CAD build for the part. Positions are in the model's coordinates, mm. A direction names the side the tool comes from. Give positions to 0.01 mm unless a question says otherwise; leave off trailing zeros. Loops run counter-clockwise (first coordinate to the right, second up) from the corner with the lowest first, then second, coordinate; pieces in that order, holes last.
Item 1: Mould opens along X. For faces 3 (the flat face through (2, 0, 182)), 4 (the flat face through (143.29, 1.57, -95.33)), 5 (the cylindrical face through (88.43, 1.61, 171.83)) say: released by +X, released by -X, zero draft, split by the parting line, or undercut.
Item 2: Saw through at A-A on z = 109. Give the cut face in (x, y) (3 decimals).
Item 3: Saw through at B-B on z = -55.5. Give the cut face in (x, y) (3 decimals).
Item 4: Saw through at C-C on y = 1.5. Give the number of separate pieces and of enclosed holes in the cut face, plus the area to 3 significant figures.
Item 5: Which spindle directions (+Z, -Z, +X, -X, +Y, -Y) get a long thin tool onto all of the face, cutting with end or side? Do faces 1 (the cylindrical face through (-123.61, 1.61, 136.65)), 2 (the flat face through (2, 3.175, 182)). Say none if no direction does.
Item 6: Probe probe 1 along Z at (x, y) = (-66.5, 1.1); probe 2 along Z at (x, y) = (30, 0.2); probe 3 along Z at (x, y) = (42.5, 0.75). List the from-to ranges inside material, lowest first.
from build123d import *

# Parameters (mm, degrees)
BOSS_EXTRUDE1_DEPTH = 3.175
CUT_EXTRUDE1_DEPTH  = 252.960239461
SKETCH4_R           = 2.159
CUT_EXTRUDE2_DEPTH  = 252.960239461


with BuildPart() as part:
    # Sketch1 → Boss-Extrude1 (new body)
    with BuildSketch(Plane(origin=(0, 0, 0), x_dir=(1, 0, 0), z_dir=(0, 1, 0))):
        Polygon((-152.4, 86.220142619), (-134.439487758, 104.180654861), (134.439487758, 104.180654861), (152.4, 86.220142619), (152.4, -182.658832897), (134.439487758, -200.619345139), (-134.439487758, -200.619345139), (-152.4, -182.658832897), align=None)
    extrude(amount=BOSS_EXTRUDE1_DEPTH)

    # Sketch2 → Cut-Extrude1 (cut, through all)
    with BuildSketch(Plane(origin=(0, 3.175, 0), x_dir=(1, 0, 0), z_dir=(0, 1, 0))):
        with BuildLine():
            Line((-76.2, 78.780654861), (76.2, 78.780654861))
            ThreePointArc((76.2, 78.780654861), (88.275474207, 75.463786622), (98.518463274, 68.259630377))
            Line((98.518463274, 68.259630377), (116.478975516, 50.299118134))
            ThreePointArc((116.478975516, 50.299118134), (123.683131761, 40.056129068), (127, 27.980654861))
            Line((127, 27.980654861), (127, -124.419345139))
            ThreePointArc((127, -124.419345139), (123.683131761, -136.494819346), (116.478975516, -146.737808413))
            Line((116.478975516, -146.737808413), (98.518463274, -164.698320655))
            ThreePointArc((98.518463274, -164.698320655), (88.275474207, -171.9024769), (76.2, -175.219345139))
            Line((76.2, -175.219345139), (-76.2, -175.219345139))
            ThreePointArc((-76.2, -175.219345139), (-88.275474207, -171.9024769), (-98.518463274, -164.698320655))
            Line((-98.518463274, -164.698320655), (-116.478975516, -146.737808413))
            ThreePointArc((-116.478975516, -146.737808413), (-123.683131761, -136.494819346), (-127, -124.419345139))
            Line((-127, -124.419345139), (-127, 27.980654861))
            ThreePointArc((-127, 27.980654861), (-123.683131761, 40.056129068), (-116.478975516, 50.299118134))
            Line((-116.478975516, 50.299118134), (-98.518463274, 68.259630377))
            ThreePointArc((-98.518463274, 68.259630377), (-88.275474207, 75.463786622), (-76.2, 78.780654861))
        make_face()
    extrude(amount=-CUT_EXTRUDE1_DEPTH, mode=Mode.SUBTRACT)

    # Sketch4 → Cut-Extrude2 (cut, through all)
    with BuildSketch(Plane(origin=(0, 3.175, 0), x_dir=(1, 0, 0), z_dir=(0, 1, 0))):
        with Locations(Location((0, 92.750654861, 0), (0, 0, 270))):
            Circle(SKETCH4_R)
        with Locations(Location((-44.45, 92.750654861, 0), (0, 0, 270))):
            Circle(SKETCH4_R)
        with Locations(Location((44.45, 92.750654861, 0), (0, 0, 270))):
            Circle(SKETCH4_R)
        with Locations(Location((-22.225, 92.750654861, 0), (0, 0, 270))):
            Circle(SKETCH4_R)
        with Locations(Location((22.225, 92.750654861, 0), (0, 0, 270))):
            Circle(SKETCH4_R)
        with Locations(Location((-140.97, -48.219345139, 0), (0, 0, 270))):
            Circle(SKETCH4_R)
        with Locations(Location((-140.97, -25.994345139, 0), (0, 0, 270))):
            Circle(SKETCH4_R)
        with Locations(Location((-140.97, -3.769345139, 0), (0, 0, 270))):
            Circle(SKETCH4_R)
        with Locations(Location((140.97, -48.219345139, 0), (0, 0, 270))):
            Circle(SKETCH4_R)
        with Locations(Location((140.97, -25.994345139, 0), (0, 0, 270))):
            Circle(SKETCH4_R)
        with Locations(Location((140.97, -3.769345139, 0), (0, 0, 270))):
            Circle(SKETCH4_R)
        with Locations(Location((140.97, -92.669345139, 0), (0, 0, 90))):
            Circle(SKETCH4_R)
        with Locations(Location((140.97, -70.444345139, 0), (0, 0, 90))):
            Circle(SKETCH4_R)
        with Locations(Location((-140.97, -92.669345139, 0), (0, 0, 90))):
            Circle(SKETCH4_R)
        with Locations(Location((-140.97, -70.444345139, 0), (0, 0, 90))):
            Circle(SKETCH4_R)
        with Locations(Location((22.225, -189.189345139, 0), (0, 0, 90))):
            Circle(SKETCH4_R)
        with Locations(Location((-22.225, -189.189345139, 0), (0, 0, 90))):
            Circle(SKETCH4_R)
        with Locations(Location((44.45, -189.189345139, 0), (0, 0, 90))):
            Circle(SKETCH4_R)
        with Locations(Location((-44.45, -189.189345139, 0), (0, 0, 90))):
            Circle(SKETCH4_R)
        with Locations(Location((0, -189.189345139, 0), (0, 0, 90))):
            Circle(SKETCH4_R)
        with Locations(Location((-66.675, 92.750654861, 0), (0, 0, 270))):
            Circle(SKETCH4_R)
        with Locations(Location((66.675, 92.750654861, 0), (0, 0, 270))):
            Circle(SKETCH4_R)
        with Locations(Location((-140.97, 18.455654861, 0), (0, 0, 270))):
            Circle(SKETCH4_R)
        with Locations(Location((140.97, 18.455654861, 0), (0, 0, 270))):
            Circle(SKETCH4_R)
        with Locations(Location((140.97, -114.894345139, 0), (0, 0, 90))):
            Circle(SKETCH4_R)
        with Locations(Location((66.675, -189.189345139, 0), (0, 0, 90))):
            Circle(SKETCH4_R)
        with Locations(Location((-66.675, -189.189345139, 0), (0, 0, 90))):
            Circle(SKETCH4_R)
        with Locations(Location((-140.97, -114.894345139, 0), (0, 0, 90))):
            Circle(SKETCH4_R)
        with Locations(Location((-140.97, -137.119345139, 0), (0, 0, 270))):
            Circle(SKETCH4_R)
        with Locations(Location((-140.97, 40.680654861, 0), (0, 0, 90))):
            Circle(SKETCH4_R)
        with Locations(Location((140.97, 40.680654861, 0), (0, 0, 270))):
            Circle(SKETCH4_R)
        with Locations(Location((140.97, -137.119345139, 0), (0, 0, 90))):
            Circle(SKETCH4_R)
    extrude(amount=-CUT_EXTRUDE2_DEPTH, mode=Mode.SUBTRACT)


solid = part.part
Results below:
1. face 3: zero draft
1. face 4: released by +X
1. face 5: undercut
2. outline: (-152.4, 0) - (-127, 0) - (-127, 3.175) - (-152.4, 3.175) - close; (127, 0) - (152.4, 0) - (152.4, 3.175) - (127, 3.175) - close
3. outline: (-152.4, 0) - (-111.278, 0) - (-111.278, 3.175) - (-152.4, 3.175) - close; (111.278, 0) - (152.4, 0) - (152.4, 3.175) - (111.278, 3.175) - close
4. separate pieces: 1
4. enclosed holes: 33
4. area: 30,500 mm2
5. face 1: +Y, -Y
5. face 2: +Z, -Z, +X, -X, +Y
6. probe 1: z = -104.18 to -94.9, -90.6 to -78.78, 175.22 to 187.04, 191.34 to 200.62
6. probe 2: z = -104.18 to -78.78, 175.22 to 200.62
6. probe 3: z = -104.18 to -93.68, -91.82 to -78.78, 175.22 to 188.26, 190.12 to 200.62
